Check sheet for the modelled part. Datum: model origin and axes. Units: mm. Face numbers are marked on the shaded views. A direction names the side the tool comes from. Give positions to 0.01 mm unless a question says otherwise; leave off trailing zeros. Order: outer loops, then holes, each group sorted by start corner. A loop starts at its lowest first (then second) coordinate and runs counter-clockwise, first axis right, second up. Notation, with made-up numbers: (80.5, 44) -> (96.5, 44) arc R11 cw to (96.5, 49) -> close; hole circle Ø7 at (41.5, -30). An arc over 180 degrees is marked (long way). Write each question's results on one line, items separated by ' | '.
from build123d import *

# Parameters (mm, degrees)
BOSS_EXTRUDE2_DEPTH = 10
SKETCH3_R           = 2.6
CUT_EXTRUDE1_DEPTH  = 34.541019662
FILLET1_R           = 2
CUT_EXTRUDE2_DEPTH  = 27.515325757
FILLET2_R           = 0.5


with BuildPart() as part:
    # Sketch2 → Boss-Extrude2 (new body)
    with BuildSketch(Plane.XY):
        with BuildLine():
            Line((9.5, -10.75), (9.5, -3.279100486))
            ThreePointArc((9.5, -3.279100486), (0, 10.05), (-9.5, -3.279100486))
            Line((-9.5, -3.279100486), (-9.5, -10.75))
            Line((-9.5, -10.75), (-20, -10.75))
            Line((-20, -10.75), (-20, 14.25))
            Line((-20, 14.25), (20, 14.25))
            Line((20, 14.25), (20, -10.75))
            Line((20, -10.75), (9.5, -10.75))
        make_face()
    extrude(amount=BOSS_EXTRUDE2_DEPTH)

    # Sketch3 → Cut-Extrude1 (cut, through all)
    with BuildSketch(Plane.XZ.offset(10.75)):
        with Locations((-14.75, 5)):
            Circle(SKETCH3_R)
        with Locations((14.75, 5)):
            Circle(SKETCH3_R)
    extrude(amount=-CUT_EXTRUDE1_DEPTH, mode=Mode.SUBTRACT)

    # Fillet1
    fillet1_edges = [part.edges().sort_by_distance(p)[0] for p in [
        (20, 1.75, 10),
        (-20, 1.75, 10),
        (-20, 1.75, 0),
        (20, 1.75, 0),
    ]]
    fillet(fillet1_edges, radius=FILLET1_R)

    # Sketch4 → Cut-Extrude2 (cut, through all)
    with BuildSketch(Plane.XY.offset(10)):
        Polygon((-9.5, -10.75), (-9.5, -3.279100486), (-10.5, -10.75), align=None)
        Polygon((9.5, -10.75), (9.5, -3.279100486), (10.5, -10.75), align=None)
    extrude(amount=-CUT_EXTRUDE2_DEPTH, mode=Mode.SUBTRACT)

    # Fillet2
    fillet2_edges = [part.edges().sort_by_distance(p)[0] for p in [
        (-10, -7.014550243, 0),
        (-10, -7.014550243, 10),
        (10, -7.014550243, 0),
        (10, -7.014550243, 10),
    ]]
    fillet(fillet2_edges, radius=FILLET2_R)


solid = part.part
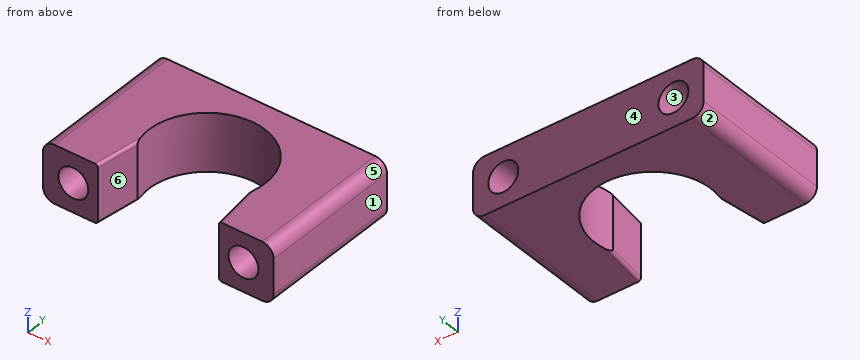
1. Section check D-D on y = 10.75. Record the cut outline in (x, z), then the cut area to 3 significant figures.
Verdict:
outline: (-20, 2) arc R2 ccw to (-18, 0) -> (18, 0) arc R2 ccw to (20, 2) -> (20, 8) arc R2 ccw to (18, 10) -> (-18, 10) arc R2 ccw to (-20, 8) -> close; hole circle Ø5.2 at (-14.75, 5); hole circle Ø5.2 at (14.75, 5) | area: 354 mm^2
2. Section check C-C on z = 7. Record the cut outline in (x, y).
Verdict:
outline: (-20, -10.75) -> (-16.41, -10.75) -> (-16.41, 14.25) -> (-20, 14.25) -> close; (-13.09, -10.75) -> (-10.5, -10.75) -> (-9.5, -3.28) arc R10.05 cw (long way) to (9.5, -3.28) -> (10.5, -10.75) -> (13.09, -10.75) -> (13.09, 14.25) -> (-13.09, 14.25) -> close; (16.41, -10.75) -> (20, -10.75) -> (20, 14.25) -> (16.41, 14.25) -> close
3. Access from +Z, -Z, +X, -X, +Y, -Y to the whole of each face (thin tool, end or side, straight path). Record for the marked faces 5 and 6.
Verdict:
face 5: +Z, +X, +Y, -Y | face 6: +Z, -Z, -Y
4. Mould release check, pull along X, two halves, no side actions. Record for the marked faces 1, 2, 3 and 4: +X half, -X half, draft (parallel to the pull), parting line (faces both ways), or undercut.
Verdict:
face 1: +X half | face 2: -X half | face 3: undercut | face 4: draft
5. Material ranges on probe 1 along Z at (x, y) = (-14.75, 8); probe 2 along X at (y, z) = (-1.5, 5.25); probe 3 along X at (y, z) = (8.75, 5.75), recorded low to high. Write a range as from..to.
Verdict:
probe 1: z = 0..2.4, 7.6..10 | probe 2: x = -20..-17.34, -12.16..-9.94, 9.94..12.16, 17.34..20 | probe 3: x = -20..-17.24, -12.26..-4.94, 4.94..12.26, 17.24..20
6. Section check B-B on x = -14.75. Record the cut outline in (y, z), then the cut area to 3 significant figures.
Verdict:
outline: (-10.75, 0) -> (14.25, 0) -> (14.25, 2.4) -> (-10.75, 2.4) -> close; (-10.75, 7.6) -> (14.25, 7.6) -> (14.25, 10) -> (-10.75, 10) -> close | area: 120 mm^2
7. Section check A-A on y = -0.5. Record the cut outline in (x, z), then the cut area to 3 significant figures.
Verdict:
outline: (-20, 2) arc R2 ccw to (-18, 0) -> (-10.04, 0) -> (-10.04, 10) -> (-18, 10) arc R2 ccw to (-20, 8) -> close; (10.04, 0) -> (18, 0) arc R2 ccw to (20, 2) -> (20, 8) arc R2 ccw to (18, 10) -> (10.04, 10) -> close; hole circle Ø5.2 at (-14.75, 5); hole circle Ø5.2 at (14.75, 5) | area: 153 mm^2
